Geometry: see drawing. Coordinates: mm, zero at the bounding-box minimum. Round coordinates to 2 decimals unless told otherwise and drop trailing zeros. Loops run counter-clockwise (first coordinate to the right, second up) from the corner with the lowest first, then second, coordinate; pieces in that order, holes last.
(1) Line query: line 1 (X direction, y = 11, z = 368); line 2 (Z direction, x = 327.5, y = 5). Output: solid intervals per line, ascending.
(2) First-contact query: pin 1 Ø6 at (y, z) = (39.5, 118.5) entering from -X; pin 2 Ø6 at (x, y) = (492, 28.5) entering from -Z; pin 3 Ø1.5 at (x, y) = (278.5, 9) entering from +Z. Flat tips, straight axial feed; report the tip coordinate or a pass-through.
(3) Cut plane A-A, the plane x = 98. Output: boundary loops of the cut face in (y, z).
(4) Cut plane C-C, the plane y = 29. Output: boundary loops of the cut face in (x, z).
(5) Cut plane B-B, the plane z = 368.3. Output: boundary loops of the cut face in (x, y), and give its area (3 significant figures).
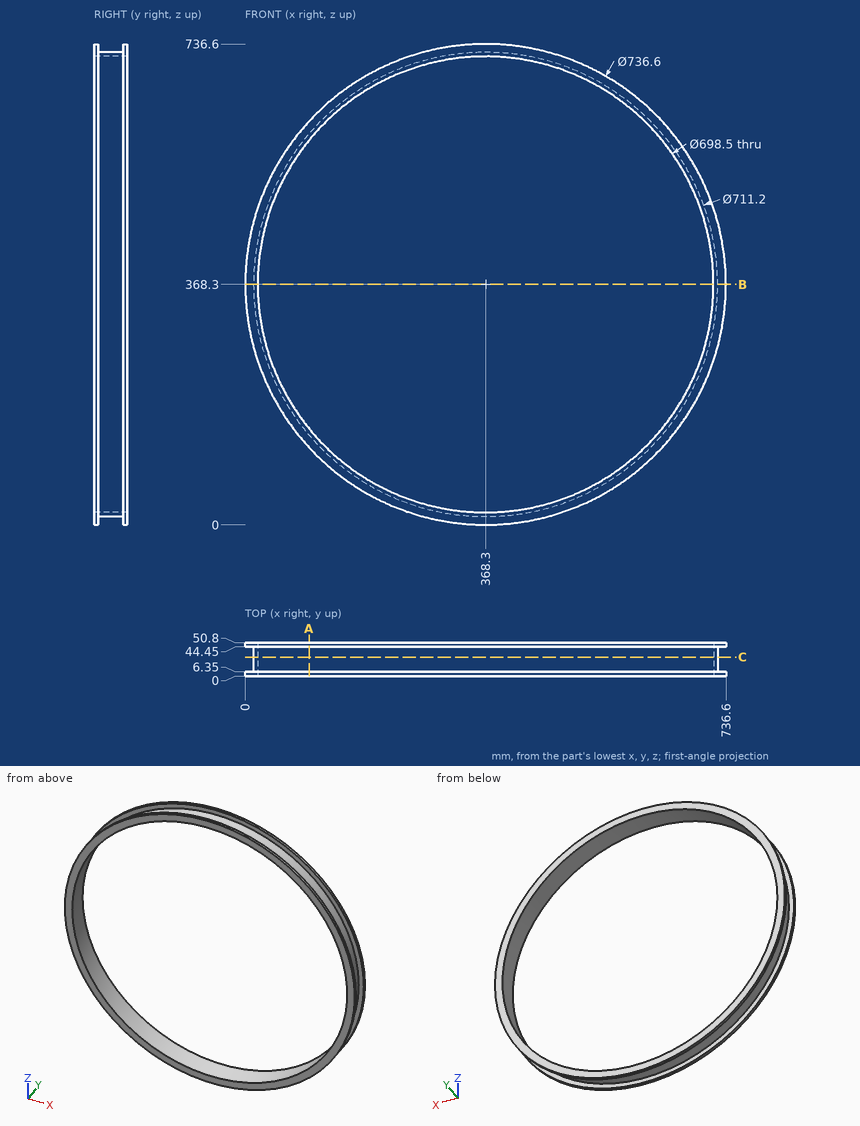
Reported:
1. line 1: x = 12.7 to 19.05, 717.55 to 723.9
1. line 2: z = 2.27 to 21.44, 715.16 to 734.33
2. pin 1: stops at x = 112.29
2. pin 2: stops at z = 33.81
2. pin 3: stops at z = 712.57
3. outline: (0, 118.13) - (6.35, 118.13) - (6.35, 137.24) - (44.45, 137.24) - (44.45, 118.13) - (50.8, 118.13) - (50.8, 147.14) - (0, 147.14) - close; (0, 589.46) - (50.8, 589.46) - (50.8, 618.47) - (44.45, 618.47) - (44.45, 599.36) - (6.35, 599.36) - (6.35, 618.47) - (0, 618.47) - close
4. outline: circle Ø711.2 at (368.3, 368.3); hole circle Ø698.5 at (368.3, 368.3)
5. outline: (0, 0) - (19.05, 0) - (19.05, 50.8) - (0, 50.8) - (0, 44.45) - (12.7, 44.45) - (12.7, 6.35) - (0, 6.35) - close; (717.55, 0) - (736.6, 0) - (736.6, 6.35) - (723.9, 6.35) - (723.9, 44.45) - (736.6, 44.45) - (736.6, 50.8) - (717.55, 50.8) - close
5. area: 968 mm2
